Design review of the part shown in the three views and the two pictorial views. Dimensions are in mm from the part's minimum x, y and z. Coordinates: 2 decimals unless noted, no trailing zeros. Write each loop counter-clockwise with the first axis right and the second up, starting at its lowest first coordinate (ties: lowest second). Pieces come first, ordered by that corner, then holes. Notation, with made-up numbers: (-20.75, 6) -> (27.25, 6) arc R23 ccw to (27.25, 39) -> close; hole circle Ø9 at (79, 73). An arc over 180 degrees is marked (long way). Answer in a Markdown table with one row per item. Add a question column.
Item 1: Draft analysis for pull direction Z (two halves, no side actions). For the marked faces 1 and 2, state which applies: released by +Z, released by -Z, zero draft, split by the parting line, or undercut.
Item 2: Take a section at B-B, the plane x = 10. Write out the cut boundary in (y, z), and give its area (3 significant figures).
Item 3: Clearance check with flat-ended pins moving along their axes: P1, Ø2.5, axis at y = 131.5, z = 2, coming from the +X side; P2, Ø1.5, axis at x = 2, z = 3, coming from the +Y side; P3, Ø1.5, axis at x = 10.5, z = 3, coming from the +Y side. State where each tip first meets the part, or that it passes through.
Item 4: Take a section at C-C, the plane y = 52.5. Write out the cut boundary in (x, z), and give its area (3 significant figures).
Item 5: To check wall thickness, follow line 1 (Y direction, x = 4, z = 0.35); line 2 (X direction, y = 46, z = 4); line 3 (Y direction, x = 30, z = 2.1). State the ranges of each line that lie inside material, in increasing order.
Item 6: Take a section at A-A, the plane z = 1.9. Write out the cut boundary in (x, y), and give its area (3 significant figures).
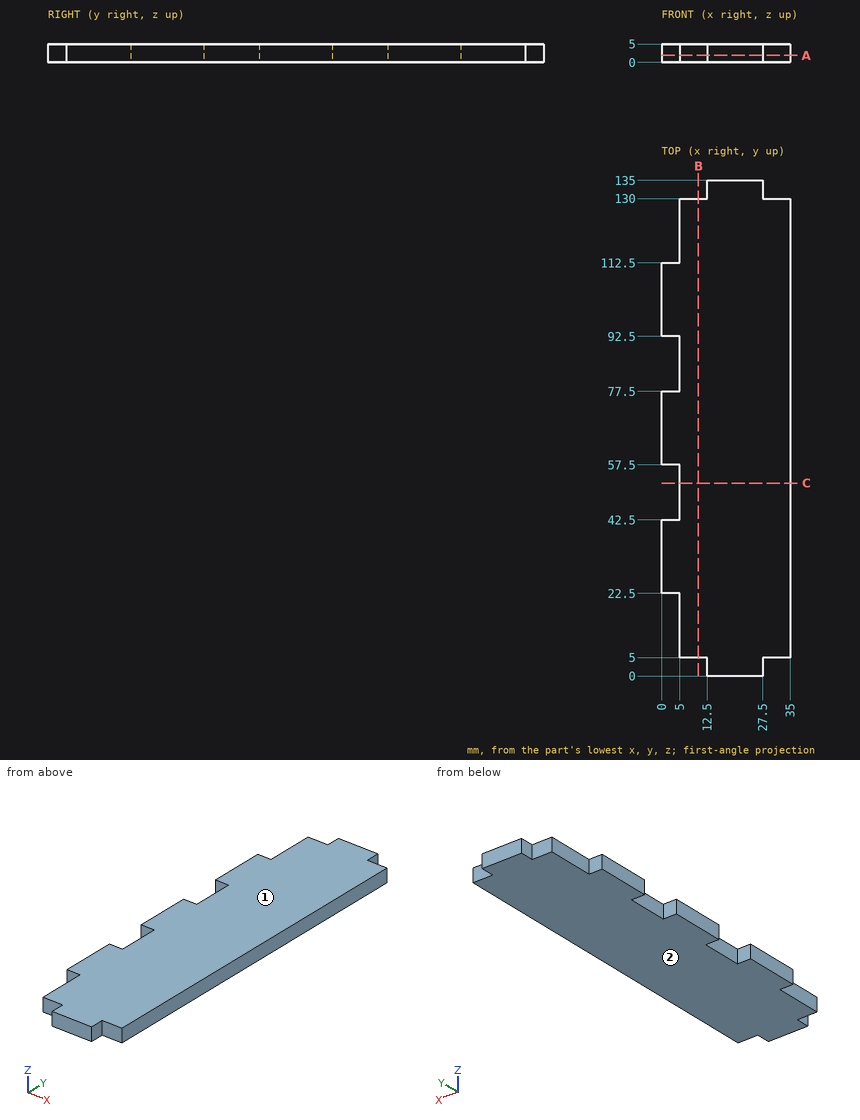
Answers:
| question | item | result |
|---|---|---|
| 1 | face 1 | released by +Z |
| 1 | face 2 | released by -Z |
| 2 | outline | (5, 0) -> (130, 0) -> (130, 5) -> (5, 5) -> close |
| 2 | area | 625 mm^2 |
| 3 | P1 | stops at x = 27.5 |
| 3 | P2 | stops at y = 112.5 |
| 3 | P3 | stops at y = 130 |
| 4 | outline | (5, 0) -> (35, 0) -> (35, 5) -> (5, 5) -> close |
| 4 | area | 150 mm^2 |
| 5 | line 1 | y = 22.5 to 42.5, 57.5 to 77.5, 92.5 to 112.5 |
| 5 | line 2 | x = 5 to 35 |
| 5 | line 3 | y = 5 to 130 |
| 6 | outline | (0, 22.5) -> (5, 22.5) -> (5, 5) -> (12.5, 5) -> (12.5, 0) -> (27.5, 0) -> (27.5, 5) -> (35, 5) -> (35, 130) -> (27.5, 130) -> (27.5, 135) -> (12.5, 135) -> (12.5, 130) -> (5, 130) -> (5, 112.5) -> (0, 112.5) -> (0, 92.5) -> (5, 92.5) -> (5, 77.5) -> (0, 77.5) -> (0, 57.5) -> (5, 57.5) -> (5, 42.5) -> (0, 42.5) -> close |
| 6 | area | 4,200 mm^2 |
